Design review of the part built by this model. Coordinates are the model's own, in mm. Coordinates: 2 decimals unless noted, no trailing zeros. Loops run counter-clockwise (first coordinate to the right, second up) from the corner with the lowest first, then second, coordinate; pieces in that order, holes last. Notation, with made-up numbers: (31.25, -21) -> (64.25, -21) arc R24 ccw to (64.25, -1) -> close; hole circle Ø1 at (47, 82.25). An arc over 180 degrees is marked (long way). Use one line per item in the form item = value. Start each with the question number.
1. For pin 1 (1 mm diameter, centred on y = 0, z = -17, fed in from +X); pin 2 (4 mm diameter, centred on x = 0, z = 7, fed in from +Y); pin 3 (1 mm diameter, centred on x = 13.5, y = 0, fed in from -Z), all flat-tipped, find the tip position at first contact; note any pin that passes through.
2. The part is to be moulded in two halves that separate along Z. For faces 1 (the face through (12.246, 0.028, -6.79)), 2 (the face through (0.07, -0.03, 5.4)), 3 (the face through (-5, -2, -1)), say which applies: released by +Z, released by -Z, zero draft, split by the parting line, or undercut.
3. Consider section C-C (z = 10). State the section outline as (x, y) points.
4. Consider section B-B (y = -1.3). State the section outline as (x, z) points.
5. Consider section A-A (x = 0). State the section outline as (y, z) points.
6. Consider section D-D (z = -7). State the section outline as (x, y) points, then the cut area to 3 significant figures.
7. Wall thickness on line 1 (X direction, y = 1.2, z = 10); line 2 (X direction, y = -0.6, z = 6); line 3 (X direction, y = 0.75, z = -7): over which ranges is each line inside the solid? List them lowest first. Write a range as from..to.
from build123d import *

# Parameters (mm, degrees)
SKETCH_2_R      = 1.6
SKETCH_2_R_2    = 4.5
EXTRUDE_1_DEPTH = 2


with BuildPart() as part:
    # 草图2 → 凸台-拉伸1 (new, symmetric)
    with BuildSketch(Plane(origin=(0, 0, 0), x_dir=(1, 0, 0), z_dir=(0, 1, 0))):
        with BuildLine():
            Line((-3.464101615, 22), (-20.784609691, -8))
            ThreePointArc((-20.784609691, -8), (-20.784609691, -12), (-17.320508076, -14))
            Line((-17.320508076, -14), (17.320508076, -14))
            ThreePointArc((17.320508076, -14), (20.784609691, -12), (20.784609691, -8))
            Line((20.784609691, -8), (3.464101615, 22))
            ThreePointArc((3.464101615, 22), (0, 24), (-3.464101615, 22))
        make_face()
        with Locations(Location((0, 7, 0), (0, 0, 270))):
            Circle(SKETCH_2_R, mode=Mode.SUBTRACT)
        with Locations(Location((0, -7, 0), (0, 0, 270))):
            Circle(SKETCH_2_R, mode=Mode.SUBTRACT)
        with Locations(Location((0, 20, 0), (0, 0, 270))):
            Circle(SKETCH_2_R, mode=Mode.SUBTRACT)
        with Locations(Location((17.320508076, -10, 0), (0, 0, 270))):
            Circle(SKETCH_2_R, mode=Mode.SUBTRACT)
        with Locations(Location((-17.320508076, -10, 0), (0, 0, 270))):
            Circle(SKETCH_2_R, mode=Mode.SUBTRACT)
        with Locations(Location((0, 0, 0), (0, 0, 270))):
            Circle(SKETCH_2_R_2, mode=Mode.SUBTRACT)
    extrude(amount=EXTRUDE_1_DEPTH, both=True)


solid = part.part
Geometry check:
q1.pin_1 = 6.64
q1.pin_2 = 2
q1.pin_3 = -5.48
q2.face_1 = released by -Z
q2.face_2 = undercut
q2.face_3 = zero draft
q3.outline = (-21.32, -2) -> (-18.92, -2) -> (-18.92, 2) -> (-21.32, 2) -> close; (-15.72, -2) -> (15.72, -2) -> (15.72, 2) -> (-15.72, 2) -> close; (18.92, -2) -> (21.32, -2) -> (21.32, 2) -> (18.92, 2) -> close
q4.outline = (-20.78, 8) -> (-3.46, -22) arc R4 ccw to (3.46, -22) -> (20.78, 8) arc R4 ccw to (17.32, 14) -> (-17.32, 14) arc R4 ccw to start; hole circle Ø3.2 at (-17.32, 10); hole circle Ø9 at (0, 0); hole circle Ø3.2 at (0, -20); hole circle Ø3.2 at (0, -7); hole circle Ø3.2 at (0, 7); hole circle Ø3.2 at (17.32, 10)
q5.outline = (-2, -24) -> (2, -24) -> (2, -21.6) -> (-2, -21.6) -> close; (-2, -18.4) -> (2, -18.4) -> (2, -8.6) -> (-2, -8.6) -> close; (-2, -5.4) -> (2, -5.4) -> (2, -4.5) -> (-2, -4.5) -> close; (-2, 4.5) -> (2, 4.5) -> (2, 5.4) -> (-2, 5.4) -> close; (-2, 8.6) -> (2, 8.6) -> (2, 14) -> (-2, 14) -> close
q6.outline = (-12.12, -2) -> (-1.6, -2) -> (-1.6, 2) -> (-12.12, 2) -> close; (1.6, -2) -> (12.12, -2) -> (12.12, 2) -> (1.6, 2) -> close
q6.area = 84.2 mm²
q7.line_1 = -21.32..-18.92, -15.72..15.72, 18.92..21.32
q7.line_2 = -19.63..-1.25, 1.25..19.63
q7.line_3 = -12.12..-1.6, 1.6..12.12
